Autodesk Inventor part; units mm, degrees
ref_plane "YZ Plane" through (0, 0, 0) normal (1, 0, 0) x (0, 1, 0)
ref_plane "XZ Plane" through (0, 0, 0) normal (0, 1, 0) x (-1, 0, 0)
ref_plane "XY Plane" through (0, 0, 0) normal (0, 0, 1) x (1, 0, 0)
sketch "Sketch1" plane through (0, 0, 0) normal (0, 0, 1) x (1, 0, 0)
  line L0 (0, 14.2875) -> (6.35, 14.2875)
  line L1 (6.35, 14.2875) -> (6.35, 15.2875)
  line L2 (6.35, 15.2875) -> (7.9248, 15.2875)
  line L3 (7.9248, 15.2875) -> (7.9248, 6.35)
  line L4 (7.9248, 6.35) -> (0, 6.35)
  line L5 (0, 6.35) -> (0, 14.2875)
  line L6 (0, 0) -> (7.9248, 0)
  line L7 (0, 11.85) -> (1, 11.85)
  line L8 (1, 11.85) -> (1, 8.85)
  line L9 (1, 8.85) -> (0, 8.85)
  line L10 (0, 8.85) -> (0, 11.85)
  line L11 (7.9248, 8.85) -> (6.9248, 8.85)
  line L12 (6.9248, 8.85) -> (6.9248, 11.85)
  line L13 (6.9248, 11.85) -> (7.9248, 11.85)
  line L14 (7.9248, 11.85) -> (7.9248, 8.85)
  dimension "d0" = 7.9248
  dimension "d2" = 12.7
  dimension "d3" = 28.575
  dimension "d4" = 1.5748
  dimension "d5" = 1
  dimension "d7" = 1
  dimension "d8" = 3
  dimension "d9" = 2.5
revolve "Revolution1" add sketch "Sketch1" angle 360 about axis through (0, 0, 0) along (1, 0, 0) contours L0 L1 L2 L3 L13 L12 L11 L4 L5 L9 L8 L7
properties part number "RoundBearing-1-2-inch"
Work out the finished part from the listing and answer in its coordinate system (mm). A direction names the side the tool comes from. Give positions to 0.01 mm unless a question says otherwise; leave off trailing zeros. Loops run counter-clockwise (first coordinate to the right, second up) from the corner with the lowest first, then second, coordinate; pieces in that order, holes last. Notation, with made-up numbers: (-26, -2) -> (23, -2) arc R28 ccw to (23, 20) -> close; hole circle Ø3 at (76.5, 64). An arc over 180 degrees is marked (long way). Use a Markdown table: item, result. Add a question column.
1) The part is cut by section A-A, the plane y = 0. Determine the outline of the cut face in (x, z).
2) Which of the six approach directions +Z, -Z, +X, -X, +Y, -Y give full straight-line access (tool end or side, diameter ignored) to faces 4 (the cylindrical face through (3.91, -1.38, 6.2)), 5 (the cylindrical face through (7.432, 11.303, 3.559)), 6 (the flat face through (6.35, 9, -11.3))?
3) The part is cut by section D-D, the plane y = -7. Determine the outline of the cut face in (x, z).
4) Consider line 1 along Z through (x, y) = (0.3, 0); line 2 along Z through (x, y) = (7.4, 0); line 3 along Z through (x, y) = (7, 6.5). Determine where each line is inside the solid, lowest interval first.
5) For a pull along Z with two mould halves and no side action, classify faces 1 (the flat face through (0, 4, -6)), 2 (the flat face through (1, -9, -1)), 3 (the cylindrical face through (7.148, 14.582, 4.592)) as +Z half, -Z half, draft (parallel to the pull), parting line (faces both ways), or undercut.
6) Each of these flat-tipped pins is pushed along its axis until it touches: P1, Ø9, axis at y = -5, z = -2, coming from the -X side; P2, Ø7.5, axis at y = 0, z = 0, coming from the +X side. Where does it stop, or does it pass through?
Reported:
| question | item | result |
|---|---|---|
| 1 | outline | (0, -14.29) -> (6.35, -14.29) -> (6.35, -15.29) -> (7.92, -15.29) -> (7.92, -11.85) -> (6.92, -11.85) -> (6.92, -8.85) -> (7.92, -8.85) -> (7.92, -6.35) -> (0, -6.35) -> (0, -8.85) -> (1, -8.85) -> (1, -11.85) -> (0, -11.85) -> close; (0, 6.35) -> (7.92, 6.35) -> (7.92, 8.85) -> (6.92, 8.85) -> (6.92, 11.85) -> (7.92, 11.85) -> (7.92, 15.29) -> (6.35, 15.29) -> (6.35, 14.29) -> (0, 14.29) -> (0, 11.85) -> (1, 11.85) -> (1, 8.85) -> (0, 8.85) -> close |
| 2 | face 4 | +X, -X |
| 2 | face 5 | +X |
| 2 | face 6 | -X |
| 3 | outline | (0, -12.46) -> (6.35, -12.46) -> (6.35, -13.59) -> (7.92, -13.59) -> (7.92, -9.56) -> (6.92, -9.56) -> (6.92, -5.42) -> (7.92, -5.42) -> (7.92, 5.42) -> (6.92, 5.42) -> (6.92, 9.56) -> (7.92, 9.56) -> (7.92, 13.59) -> (6.35, 13.59) -> (6.35, 12.46) -> (0, 12.46) -> (0, 9.56) -> (1, 9.56) -> (1, 5.42) -> (0, 5.42) -> (0, -5.42) -> (1, -5.42) -> (1, -9.56) -> (0, -9.56) -> close |
| 4 | line 1 | z = -14.29 to -11.85, -8.85 to -6.35, 6.35 to 8.85, 11.85 to 14.29 |
| 4 | line 2 | z = -15.29 to -11.85, -8.85 to -6.35, 6.35 to 8.85, 11.85 to 15.29 |
| 4 | line 3 | z = -13.84 to -9.91, -6.01 to 6.01, 9.91 to 13.84 |
| 5 | face 1 | draft |
| 5 | face 2 | undercut |
| 5 | face 3 | parting line |
| 6 | P1 | stops at x = 0 |
| 6 | P2 | passes through |
